Geometry: see drawing. Coordinates: mm, zero at the bounding-box minimum. Coordinates: 2 decimals unless noted, no trailing zeros. Order: outer loops, then holes, each group sorted by start corner. A loop starts at its lowest first (then second) coordinate and runs counter-clockwise, first axis right, second up.
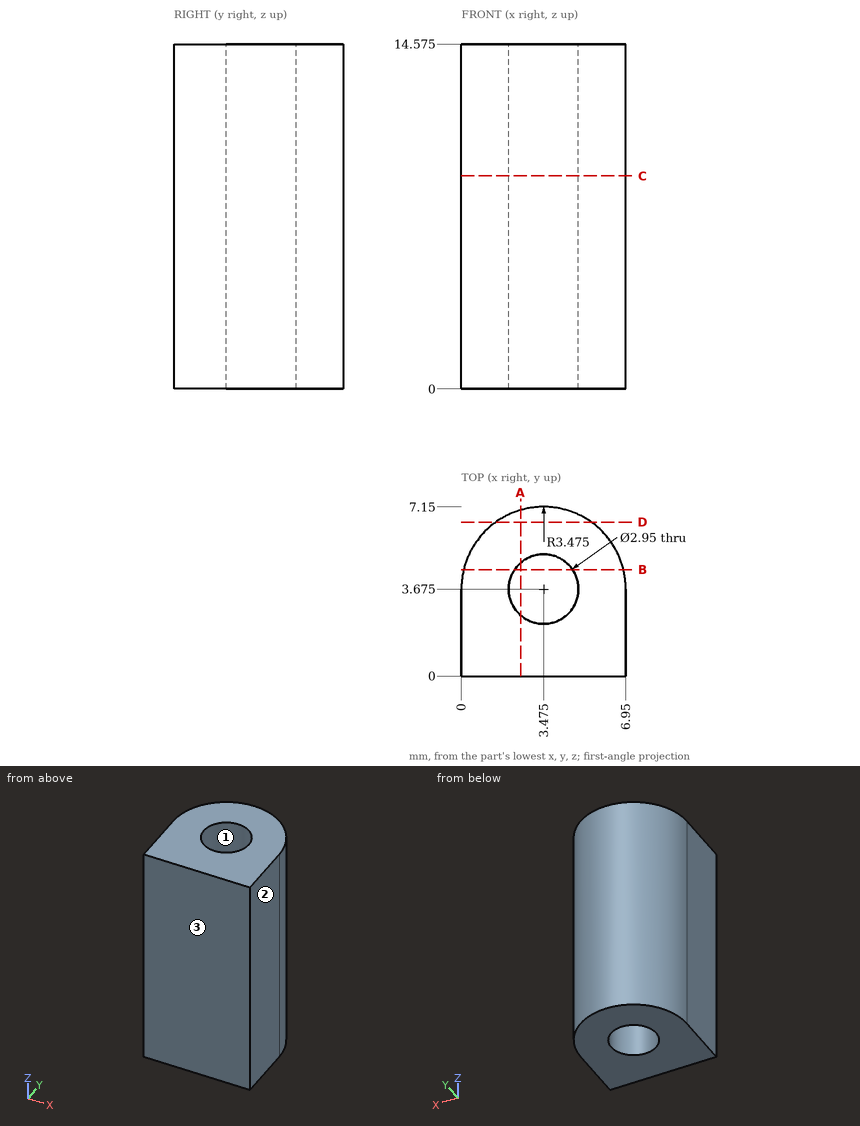
Item 1: Ray query, probe 1 along Y at (x, z) = (4.25, 6.25); probe 2 along Y at (x, z) = (3.25, 7); probe 3 along Y at (x, z) = (6.25, 3.5). Return the intervals inside material, ascending.
Response values:
probe 1: y = 0 to 2.42, 4.93 to 7.06
probe 2: y = 0 to 2.22, 5.13 to 7.14
probe 3: y = 0 to 5.77
Item 2: Cut plane B-B on y = 4.5. Return loops of the section in (x, z) (3 decimals), then the cut area to 3 significant figures.
Response values:
outline: (0.099, 0) - (2.252, 0) - (2.252, 14.575) - (0.099, 14.575) - close; (4.698, 0) - (6.851, 0) - (6.851, 14.575) - (4.698, 14.575) - close
area: 62.8 mm2
Item 3: Cut plane A-A on x = 2.5. Return loops of the section in (y, z) (3 decimals), then the cut area to 3 significant figures.
Response values:
outline: (0, 0) - (2.568, 0) - (2.568, 14.575) - (0, 14.575) - close; (4.782, 0) - (7.01, 0) - (7.01, 14.575) - (4.782, 14.575) - close
area: 69.9 mm2
Item 4: Draft query along Y for the marked faces 1, 2 and 3. Return one class per face: pulls with the +Y half, pulls with the -Y half, needs draft (parallel to the pull), parting line crosses it, or undercut.
Response values:
face 1: undercut
face 2: needs draft
face 3: pulls with the -Y half
Item 5: Pin query (flat end, axial travel): pin 1 Ø2 at (x, z) = (1.5, 4.5) entering from +Y; pin 2 Ø2.5 at (x, y) = (3.475, 3.675) entering from -Z (3 decimals). Return the tip coordinate at first contact, or that it passes through.
Response values:
pin 1: stops at y = 7.01
pin 2: passes through
Item 6: Cut plane C-C on z = 9. Return loops of the section in (x, y) (3 decimals), then the cut area to 3 significant figures.
Response values:
outline: (0, 0) - (6.95, 0) - (6.95, 3.675) arc R3.475 ccw to (0, 3.675) - close; hole circle Ø2.95 at (3.475, 3.675)
area: 37.7 mm2
Item 7: Cut plane D-D on y = 6.5. Return loops of the section in (x, z) (3 decimals), then the cut area to 3 significant figures.
Response values:
outline: (1.451, 0) - (5.499, 0) - (5.499, 14.575) - (1.451, 14.575) - close
area: 59.0 mm2
